```python
from build123d import *

# Parameters (mm, degrees)
SKETCH_W   = 10
SKETCH_H   = 100
SKETCH_W_2 = 6
SKETCH_H_2 = 96
PAD_DEPTH  = 700


with BuildPart() as part:
    # Sketch → Pad (new body)
    with BuildSketch(Plane.YZ):
        with Locations((5, -50)):
            Rectangle(SKETCH_W, SKETCH_H)
        with Locations((5, -50)):
            Rectangle(SKETCH_W_2, SKETCH_H_2, mode=Mode.SUBTRACT)
    extrude(amount=PAD_DEPTH)


solid = part.part
```
For this review, take the finished solid that the model builds, in its own axes (mm). Round coordinates to 2 decimals unless told otherwise and drop trailing zeros. Write each loop counter-clockwise with the first axis right and the second up, starting at its lowest first coordinate (ties: lowest second). Pieces come first, ordered by that corner, then holes. Notation, with made-up numbers: (19.5, 13) - (55.5, 13) arc R22 ccw to (55.5, 43) - close; hole circle Ø4 at (-25, 4.5). An arc over 180 degrees is marked (long way). Put each result on its own line as item: value.
Q1. We need section B-B (x = 118). Give the boundary of the cut face in (y, z).
Solved:
outline: (0, -100) - (10, -100) - (10, 0) - (0, 0) - close; hole (2, -98) - (8, -98) - (8, -2) - (2, -2) - close
Q2. Insertion check: pin 1 Ø1.8 at (x, y) = (330.5, 6) entering from +Z. The pin has a flat end and moves straight along its axis. Give the tip position at first contact, or say it passes through.
Solved:
pin 1: stops at z = 0
Q3. We need section A-A (y = 3.75). Give the boundary of the cut face in (x, z), and give its area (3 significant figures).
Solved:
outline: (0, -100) - (700, -100) - (700, -98) - (0, -98) - close; (0, -2) - (700, -2) - (700, 0) - (0, 0) - close
area: 2,800 mm2
Q4. Mouldability with a two-part tool opening along Y and no side actions: class faces 1 (the face through (345, 8, -51)), 2 (the face through (345, 10, -51)), 3 (the face through (345, 0, -51)), 4 (the face through (345, 2, -51)) as released by +Y, released by -Y, zero draft, split by the parting line, or undercut.
Solved:
face 1: undercut
face 2: released by +Y
face 3: released by -Y
face 4: undercut
Q5. Wall thickness on probe 1 along Y at (x, z) = (303, -74.5); probe 2 along Z at (x, y) = (204, 5.25): over which ranges is each line inside the solid? List them lowest first.
Solved:
probe 1: y = 0 to 2, 8 to 10
probe 2: z = -100 to -98, -2 to 0
Q6. We need section C-C (z = -39.5). Give the boundary of the cut face in (x, y), and give its area (3 significant figures).
Solved:
outline: (0, 0) - (700, 0) - (700, 2) - (0, 2) - close; (0, 8) - (700, 8) - (700, 10) - (0, 10) - close
area: 2,800 mm2
